from build123d import *

# Parameters (mm, degrees)
SKETCH1_R          = 36.5125
SKETCH1_R_2        = 31.3563
BASE_EXTRUDE_DEPTH = 914.4
CUT_EXTRUDE5_DEPTH = 76.2
SKETCH4_R          = 3.9751
CUT_EXTRUDE2_DEPTH = 63.5
SKETCH5_R          = 3.9751
CUT_EXTRUDE3_DEPTH = 881.900721082


with BuildPart() as part:
    # Sketch1 → Base-Extrude (new, symmetric)
    with BuildSketch(Plane.XY):
        Circle(SKETCH1_R)
        Circle(SKETCH1_R_2, mode=Mode.SUBTRACT)
    extrude(amount=BASE_EXTRUDE_DEPTH, both=True)

    # Sketch6 → Cut-Extrude5 (cut, symmetric)
    with BuildSketch(Plane(origin=(0, 0, 0), x_dir=(0, 0, -1), z_dir=(1, 0, 0))):
        Polygon((-956.15258377, 192.708539462), (-746.964120429, -232.924753088), (-956.15258377, -232.924753088), align=None)
        Polygon((766.72941623, 192.708539462), (975.917879571, -232.924753088), (975.917879571, 192.708539462), align=None)
    extrude(amount=CUT_EXTRUDE5_DEPTH, both=True, mode=Mode.SUBTRACT)

    # Sketch4 → Cut-Extrude2 (cut, symmetric)
    with BuildSketch(Plane(origin=(0, 0, 0), x_dir=(1, 0, 0), z_dir=(0, 1, 0))):
        with Locations(Location((0, 863.6, 0), (0, 0, 270))):
            Circle(SKETCH4_R)
    extrude(amount=CUT_EXTRUDE2_DEPTH, both=True, mode=Mode.SUBTRACT)

    # Sketch5 → Cut-Extrude3 (cut, through all)
    with BuildSketch(Plane(origin=(0, 0, 0), x_dir=(1, 0, 0), z_dir=(0, 1, 0))):
        with Locations(Location((0, 827.62098982, 0), (0, 0, 90))):
            Circle(SKETCH5_R)
    extrude(amount=CUT_EXTRUDE3_DEPTH, mode=Mode.SUBTRACT)


solid = part.part
Here's how the part is built. I have some questions about the finished solid (model axes, mm). Round coordinates to 2 decimals unless told otherwise and drop trailing zeros. Order: outer loops, then holes, each group sorted by start corner. A loop starts at its lowest first (then second) coordinate and runs counter-clockwise, first axis right, second up. Notation, with made-up numbers: M 37.25,75.25 L 79.25,75.25 A26 cw 79.25,108.25 Z; hole C 83,88.25 d9. An arc over 180 degrees is marked long. Return JSON: item names as keys, results as strings. Group by question number.
1. If we mould it in two halves opening along Y, with no side actions, what happens to faces 1 (the face through (-24.883, -19.08, -12.28)), 2 (the face through (34.826, 10.967, 12.316)), 3 (the face through (29.921, -10.648, -866.674))? For each: pulls with the +Y half, pulls with the -Y half, needs draft (parallel to the pull), parting line crosses it, or undercut.
2. If we section it at A-A on y = -18.5: List the corners of the cut face in (x, z) for me.
3. If we section it at C-C on z = 521.5: List the corners of the cut face in (x, y) for me (1 decimal), then the cut area to 3 significant figures.
4. I'm going to push flat-ended pins straight in: pin 1 Ø10 at (y, z) = (-16, 572) entering from +X; pin 2 Ø1 at (x, z) = (28, 420.5) entering from +Y; pin 3 Ø5 at (x, z) = (-9.5, -303) entering from +Y. Where does each tip first touch, or does it pass through?
5. Please list where these lines run through material, in increasing order: probe 1 along X at (y, z) = (0, -194.5); probe 2 along Y at (x, z) = (1.5, -625).
6. If we section it at B-B on x = -15.5: List the corners of the cut face in (y, z) for me.
Reply:
{
 "1": {"face 1": "undercut", "face 2": "parting line crosses it", "face 3": "pulls with the +Y half"},
 "2": {"outline": "M -31.48,-870.53 L -25.32,-870.53 L -25.32,852.35 L -31.48,852.35 Z; M 25.32,-870.53 L 31.48,-870.53 L 31.48,852.35 L 25.32,852.35 Z"},
 "3": {"outline": "C 0,0 d73; hole C 0,0 d62.7", "area": "1,100 mm^2"},
 "4": {"pin 1": "x = 34.82", "pin 2": "y = 24.02", "pin 3": "y = 35.84"},
 "5": {"probe 1": "-36.51 to -31.36, 31.36 to 36.51", "probe 2": "-36.48 to -31.32, 31.32 to 36.48"},
 "6": {"outline": "M -33.06,-877.69 L -27.26,-874.84 L -27.26,848.04 L -33.06,845.19 Z; M 27.26,-848.04 L 33.06,-845.19 L 33.06,877.69 L 27.26,874.84 Z"}
}
